Part model, mm, in its own coordinate system. A direction names the side the tool comes from. Round coordinates to 2 decimals unless told otherwise and drop trailing zeros. Write each loop counter-clockwise with the first axis right and the second up, starting at its lowest first coordinate (ties: lowest second). Pieces come first, ordered by that corner, then holes.
```python
from build123d import *

# Parameters (mm, degrees)
SKETCH1_W           = 22
SKETCH1_H           = 22
SKETCH1_R           = 1.55
SKETCH1_R_2         = 8.5
BOSS_EXTRUDE1_DEPTH = 3
BOSS_EXTRUDE2_DEPTH = 3


with BuildPart() as part:
    # Sketch1 → Boss-Extrude1 (new body)
    with BuildSketch(Plane(origin=(0, 0, 0), x_dir=(1, 0, 0), z_dir=(0, 1, 0))):
        with Locations((-27.765585807, 11.176708998)):
            Rectangle(SKETCH1_W, SKETCH1_H)
        with Locations((-19.305585807, 2.716708998)):
            Circle(SKETCH1_R, mode=Mode.SUBTRACT)
        with Locations((-31.905585807, 19.716708998)):
            Circle(SKETCH1_R, mode=Mode.SUBTRACT)
        with Locations((-26.223701498, 10.648645815)):
            Circle(SKETCH1_R_2, mode=Mode.SUBTRACT)
    extrude(amount=BOSS_EXTRUDE1_DEPTH)

    # Sketch2 → Boss-Extrude2 (add)
    with BuildSketch(Plane(origin=(0, 3, 0), x_dir=(1, 0, 0), z_dir=(0, 1, 0))):
        Polygon((-38.765585807, 0.176708998), (-38.765585807, -15.991830681), (-34.011681836, -20.745734651), (-25.445380771, -12.179433585), (-29.728531303, -7.896283053), (-29.728531303, 0.176708998), align=None)
        Polygon((-38.765585807, 22.176708998), (-38.765585807, 36.389702532), (-33.427082463, 41.728205876), (-26.085708647, 34.38683206), (-29.756395555, 30.716145153), (-29.756395555, 22.176708998), align=None)
    extrude(amount=-BOSS_EXTRUDE2_DEPTH)


solid = part.part
```
Q1. Mould opens along Z. For faces 1 (the flat face through (-23, 1, -22.177)), 2 (the flat face through (-36.134, 1.521, -39.022)), 3 (the flat face through (-29.788, 1.521, 16.523)), 4 (the flat face through (-35, 0, -11)) say: +Z half, -Z half, draft (parallel to the pull), parting line (faces both ways), or undercut.
Values follow:
face 1: undercut
face 2: -Z half
face 3: +Z half
face 4: draft
Q2. Drop flat-ended pins along their axis: pin 1 (5 mm diameter, centred on x = -24, z = -6, fed in from +Y); pin 2 (0.9 mm diameter, centred on y = 1.5, z = 3.5, fed in from +X); pin 3 (0.9 mm diameter, centred on y = 2, z = -27, fed in from +X); pin 4 (1 mm diameter, centred on x = -32.5, y = 2, fed in from -Z). Give the stop position or say it passes through.
Values follow:
pin 1: passes through
pin 2: stops at x = -29.73
pin 3: stops at x = -29.76
pin 4: stops at z = -41.3
Q3. Cut at A-A on z = -16. Write the cut outline in (x, y).
Values follow:
outline: (-38.77, 0) - (-32.83, 0) - (-32.83, 3) - (-38.77, 3) - close; (-19.62, 0) - (-16.77, 0) - (-16.77, 3) - (-19.62, 3) - close
Q4. Cut at D-D on x = -32.75. Write the cut outline in (y, z), plus the area to 3 significant figures.
Values follow:
outline: (0, -41.05) - (3, -41.05) - (3, -21.02) - (0, -21.02) - close; (0, -18.42) - (3, -18.42) - (3, -16.09) - (0, -16.09) - close; (0, -5.2) - (3, -5.2) - (3, 19.48) - (0, 19.48) - close
area: 141 mm2
Q5. Cut at B-B on x = -28. Write the cut outline in (y, z), plus the area to 3 significant figures.
Values follow:
outline: (0, -36.3) - (3, -36.3) - (3, -32.47) - (0, -32.47) - close; (0, -22.18) - (3, -22.18) - (3, -18.96) - (0, -18.96) - close; (0, -2.34) - (3, -2.34) - (3, -0.18) - (0, -0.18) - close; (0, 9.62) - (3, 9.62) - (3, 14.73) - (0, 14.73) - close
area: 42.9 mm2
Q6. Cut at C-C on y = 0.5. Write the cut outline in (x, z).
Values follow:
outline: (-38.77, -36.39) - (-33.43, -41.73) - (-26.09, -34.39) - (-29.76, -30.72) - (-29.76, -22.18) - (-16.77, -22.18) - (-16.77, -0.18) - (-29.73, -0.18) - (-29.73, 7.9) - (-25.45, 12.18) - (-34.01, 20.75) - (-38.77, 15.99) - close; hole circle Ø17 at (-26.22, -10.65); hole circle Ø3.1 at (-31.91, -19.72); hole circle Ø3.1 at (-19.31, -2.72)
Q7. Which spindle directions (+Z, -Z, +X, -X, +Y, -Y) get a long thin tool onto all of the face, cutting with end or side? Do faces 5 (the flat face through (-23, 1, -0.177)), 6 (the cylindrical face through (-34.715, 1.479, -11.022)). Say none if no direction does.
Values follow:
face 5: +X, +Y, -Y
face 6: +Y, -Y
Q8. Wall check: L1, parallel to Z at x = -19.5, y = 1.4; L2, parallel to Z at x = -25.75, y = 1.95; L3, parallel to Z at x = -27, y = 0.7. Give the ranges that are in metal, low to high.
Values follow:
L1: z = -22.18 to -15.85, -5.45 to -4.25, -1.18 to -0.18
L2: z = -22.18 to -19.14, -2.16 to -0.18, 11.87 to 12.48
L3: z = -35.3 to -33.47, -22.18 to -19.11, -2.18 to -0.18, 10.62 to 13.73
